Part model, mm, in its own coordinate system. Face numbers are marked on the shaded views. Round coordinates to 2 decimals unless told otherwise and drop trailing zeros. Write each loop counter-clockwise with the first axis right and the second up, starting at its lowest first coordinate (ties: lowest second). Pieces come first, ordered by that corner, then holes.
1) Saw through at C-C on y = 7. Write the cut outline in (x, z), and give its area (3 significant figures).
2) Pull direction X, two halves, no side cores. Call the marked faces 1, 2 and 3: +X half, -X half, draft (parallel to the pull), parting line (faces both ways), or undercut.
3) Saw through at B-B on x = 0. Write the cut outline in (y, z).
4) Drill centre lines: L1, parallel to Y at x = 1, z = -0.5; L2, parallel to X at y = 10.25, z = 1.25; L3, parallel to X at y = 10.25, z = -2. Where is each one in solid material? Low to high.
5) Saw through at A-A on y = 9.5. Write the cut outline in (x, z), and give its area (3 significant figures).
6) Flat gauge pins, fed straight in: pin 1 (3 mm diameter, centred on x = 3.5, y = 9.5, fed in from -Z); pin 2 (2.5 mm diameter, centred on x = 0, y = 11, fed in from +Z); pin 3 (1 mm diameter, centred on y = 6.5, z = 1, fed in from -X). Where does each tip first touch, or does it go through?
```python
from build123d import *
from OCP.BRepFilletAPI import BRepFilletAPI_MakeChamfer

# Parameters (mm, degrees)
BOSS_EXTRUDE1_DEPTH  = 1.75
BOSS_EXTRUDE2_DEPTH  = 0.5
BOSS_EXTRUDE5_DEPTH  = 3.5
SKETCH4_R            = 3.5
BOSS_EXTRUDE7_DEPTH  = 2
SKETCH11_R           = 4.505443821
SKETCH11_R_2         = 3.5
CUT_EXTRUDE3_DEPTH   = 2
SKETCH12_R           = 3.5
CUT_EXTRUDE4_DEPTH   = 3
BOSS_EXTRUDE8_DEPTH  = 2.5
CHAMFER1_SIZE        = 0.5
CHAMFER1_SIZE2       = 0.288675135
SKETCH17_R           = 3.25
BOSS_EXTRUDE9_DEPTH  = 3
SKETCH18_R           = 1.768100224
CUT_EXTRUDE8_DEPTH   = 2.25
SKETCH20_R           = 5
BOSS_EXTRUDE10_DEPTH = 2
SKETCH21_R           = 5
BOSS_EXTRUDE11_DEPTH = 2
FILLET1_R            = 0.5
SKETCH25_R           = 4.000350088
CUT_EXTRUDE9_DEPTH   = 10
SKETCH26_R           = 4.25
BOSS_EXTRUDE12_DEPTH = 2.1


with BuildPart() as part:
    # Sketch1 → Boss-Extrude1 (new body)
    with BuildSketch(Plane(origin=(0, 0, 0), x_dir=(1, 0, 0), z_dir=(0, 1, 0))):
        Polygon((0.658179307, 0), (0.329089653, 0.57), (-0.329089653, 0.57), (-0.658179307, 0), (-0.329089653, -0.57), (0.329089653, -0.57), align=None)
    extrude(amount=BOSS_EXTRUDE1_DEPTH)

    # Sketch2 → Boss-Extrude2 (add)
    with BuildSketch(Plane(origin=(0, 1.75, 0), x_dir=(1, 0, 0), z_dir=(0, 1, 0))):
        Polygon((0.658179307, 0), (0.558124156, -0.173300605), (4.375, 0), (0.558578548, 0.172513574), align=None)
        Polygon((0, 0.197762982), (0, 0), (0, -0.198641554), (0.558124156, -0.173300605), (0.658179307, 0), (0.558578548, 0.172513574), align=None)
    extrude(amount=BOSS_EXTRUDE2_DEPTH)

    # Sketch3 → Boss-Extrude5 (add)
    with BuildSketch(Plane(origin=(0, 1.75, 0), x_dir=(1, 0, 0), z_dir=(0, 1, 0))):
        Polygon((0.658179307, 0), (0.329089653, 0.57), (-0.329089653, 0.57), (-0.658179307, 0), (-0.329089653, -0.57), (0.329089653, -0.57), align=None)
    extrude(amount=BOSS_EXTRUDE5_DEPTH)

    # Sketch4 → Boss-Extrude7 (add)
    with BuildSketch(Plane(origin=(0, 5.25, 0), x_dir=(1, 0, 0), z_dir=(0, 1, 0))):
        with Locations(Location((0, 0, 0), (0, 0, 270))):
            Circle(SKETCH4_R)
    extrude(amount=BOSS_EXTRUDE7_DEPTH)

    # Sketch11 → Cut-Extrude3 (cut)
    with BuildSketch(Plane(origin=(0, 1.75, 0), x_dir=(-1, 0, 0), z_dir=(0, -1, 0))):
        Circle(SKETCH11_R)
        with Locations(Location((0, 0, 0), (0, 0, 270))):
            Circle(SKETCH11_R_2, mode=Mode.SUBTRACT)
    extrude(amount=-CUT_EXTRUDE3_DEPTH, mode=Mode.SUBTRACT)

    # Sketch12 → Cut-Extrude4 (cut)
    with BuildSketch(Plane(origin=(0, 0, 0), x_dir=(-1, 0, 0), z_dir=(0, -1, 0))):
        with Locations(Location((0, 0, 0), (0, 0, 270))):
            Circle(SKETCH12_R)
    extrude(amount=-CUT_EXTRUDE4_DEPTH, mode=Mode.SUBTRACT)

    # Sketch16 → Boss-Extrude8 (add)
    with BuildSketch(Plane(origin=(0, 3, 0), x_dir=(-1, 0, 0), z_dir=(0, -1, 0))):
        Polygon((0.55, -0.952627944), (1.1, 0), (0.658179307, 0), (0.329089653, -0.57), (-0.329089653, -0.57), (-0.658179307, 0), (-1.1, 0), (-0.55, -0.952627944), align=None)
        Polygon((0.658179307, 0), (1.1, 0), (0.55, 0.952627944), (-0.55, 0.952627944), (-1.1, 0), (-0.658179307, 0), (-0.329089653, 0.57), (0.329089653, 0.57), align=None)
        Polygon((-0.658179307, 0), (0.658179307, 0), (0.329089653, 0.57), (-0.329089653, 0.57), align=None)
        Polygon((0.329089653, -0.57), (0.658179307, 0), (-0.658179307, 0), (-0.329089653, -0.57), align=None)
    extrude(amount=-BOSS_EXTRUDE8_DEPTH)

    # Chamfer1: one chamfer whose edges measure the first distance from different faces: ONE call of the kernel's chamfer builder (chamfer() names one face for all edges)
    chamfer1_edges_1 = [part.edges().sort_by_distance(p)[0] for p in [
        (-0.825, 5.25, -0.476313972),
    ]]
    chamfer1_side_1 = [part.faces().sort_by_distance(p)[0] for p in [
        (-0.825, 4.125, -0.476313972),
    ]]
    chamfer1_edges_2 = [part.edges().sort_by_distance(p)[0] for p in [
        (0, 5.25, -0.952627944),
    ]]
    chamfer1_side_2 = [part.faces().sort_by_distance(p)[0] for p in [
        (0, 4.125, -0.952627944),
    ]]
    chamfer1_edges_3 = [part.edges().sort_by_distance(p)[0] for p in [
        (0.825, 5.25, -0.476313972),
    ]]
    chamfer1_side_3 = [part.faces().sort_by_distance(p)[0] for p in [
        (0.825, 4.125, -0.476313972),
    ]]
    chamfer1_edges_4 = [part.edges().sort_by_distance(p)[0] for p in [
        (0.825, 5.25, 0.476313972),
    ]]
    chamfer1_side_4 = [part.faces().sort_by_distance(p)[0] for p in [
        (0.825, 4.125, 0.476313972),
    ]]
    chamfer1_edges_5 = [part.edges().sort_by_distance(p)[0] for p in [
        (0, 5.25, 0.952627944),
    ]]
    chamfer1_side_5 = [part.faces().sort_by_distance(p)[0] for p in [
        (0, 4.125, 0.952627944),
    ]]
    chamfer1_edges_6 = [part.edges().sort_by_distance(p)[0] for p in [
        (-0.825, 5.25, 0.476313972),
    ]]
    chamfer1_side_6 = [part.faces().sort_by_distance(p)[0] for p in [
        (-0.825, 4.125, 0.476313972),
    ]]
    chamfer1 = BRepFilletAPI_MakeChamfer(part.part.solid().wrapped)
    for e in chamfer1_edges_1:
        chamfer1.Add(CHAMFER1_SIZE, CHAMFER1_SIZE2, e.wrapped, chamfer1_side_1[0].wrapped)  # the first distance lies on this face
    for e in chamfer1_edges_2:
        chamfer1.Add(CHAMFER1_SIZE, CHAMFER1_SIZE2, e.wrapped, chamfer1_side_2[0].wrapped)  # the first distance lies on this face
    for e in chamfer1_edges_3:
        chamfer1.Add(CHAMFER1_SIZE, CHAMFER1_SIZE2, e.wrapped, chamfer1_side_3[0].wrapped)  # the first distance lies on this face
    for e in chamfer1_edges_4:
        chamfer1.Add(CHAMFER1_SIZE, CHAMFER1_SIZE2, e.wrapped, chamfer1_side_4[0].wrapped)  # the first distance lies on this face
    for e in chamfer1_edges_5:
        chamfer1.Add(CHAMFER1_SIZE, CHAMFER1_SIZE2, e.wrapped, chamfer1_side_5[0].wrapped)  # the first distance lies on this face
    for e in chamfer1_edges_6:
        chamfer1.Add(CHAMFER1_SIZE, CHAMFER1_SIZE2, e.wrapped, chamfer1_side_6[0].wrapped)  # the first distance lies on this face
    add(Compound.cast(chamfer1.Shape()), mode=Mode.REPLACE)

    # Sketch17 → Boss-Extrude9 (add)
    with BuildSketch(Plane(origin=(0, 3, 0), x_dir=(-1, 0, 0), z_dir=(0, -1, 0))):
        with Locations(Location((0, 0, 0), (0, 0, 90))):
            Circle(SKETCH17_R)
        Polygon((-2.995914926, 0), (-1.497957463, -2.594538434), (1.497957463, -2.594538434), (2.995914926, 0), (1.497957463, 2.594538434), (-1.497957463, 2.594538434), align=None, mode=Mode.SUBTRACT)
    extrude(amount=-BOSS_EXTRUDE9_DEPTH)

    # Sketch18 → Cut-Extrude8 (cut)
    with BuildSketch(Plane(origin=(0, 3, 0), x_dir=(-1, 0, 0), z_dir=(0, -1, 0))):
        Circle(SKETCH18_R)
    extrude(amount=-CUT_EXTRUDE8_DEPTH, mode=Mode.SUBTRACT)

    # Sketch20 → Boss-Extrude10 (add)
    with BuildSketch(Plane(origin=(0, 7.25, 0), x_dir=(1, 0, 0), z_dir=(0, 1, 0))):
        with Locations(Location((0, 0, 0), (0, 0, 270))):
            Circle(SKETCH20_R)
    extrude(amount=-BOSS_EXTRUDE10_DEPTH)

    # Sketch21 → Boss-Extrude11 (add)
    with BuildSketch(Plane(origin=(0, 7.25, 0), x_dir=(1, 0, 0), z_dir=(0, 1, 0))):
        with Locations(Location((0, 0, 0), (0, 0, 270))):
            Circle(SKETCH21_R)
    extrude(amount=BOSS_EXTRUDE11_DEPTH)

    # Fillet1
    fillet1_edges = [part.edges().sort_by_distance(p)[0] for p in [
        (0, 5.25, -5),
        (0, 9.25, -5),
    ]]
    fillet(fillet1_edges, radius=FILLET1_R)

    # Sketch25 → Cut-Extrude9 (cut)
    with BuildSketch(Plane(origin=(0, 5.25, 0), x_dir=(-1, 0, 0), z_dir=(0, -1, 0))):
        Circle(SKETCH25_R)
    extrude(amount=CUT_EXTRUDE9_DEPTH, mode=Mode.SUBTRACT)

    # Sketch26 → Boss-Extrude12 (add)
    with BuildSketch(Plane(origin=(0, 9.25, 0), x_dir=(1, 0, 0), z_dir=(0, 1, 0))):
        with Locations(Location((0, 0, 0), (0, 0, 270))):
            Circle(SKETCH26_R)
        Polygon((1.662768775, -2.88), (3.325537551, 0), (1.662768775, 2.88), (-1.662768775, 2.88), (-3.325537551, 0), (-1.662768775, -2.88), align=None, mode=Mode.SUBTRACT)
    extrude(amount=BOSS_EXTRUDE12_DEPTH)


solid = part.part
```
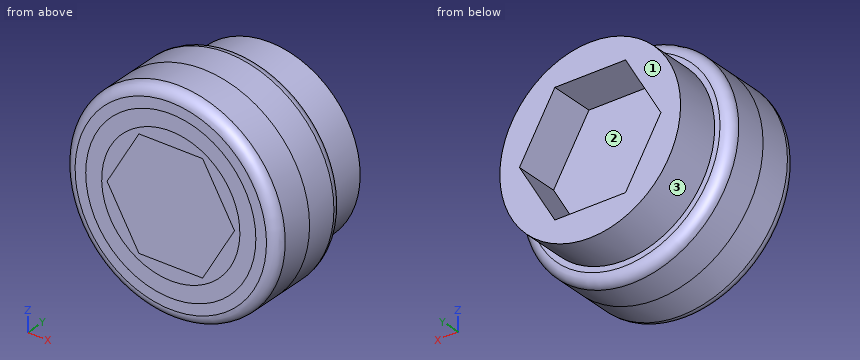
Completed:
1. outline: circle Ø10 at (0, 0)
1. area: 78.5 mm2
2. face 1: draft
2. face 2: undercut
2. face 3: parting line
3. outline: (5.25, -4.5) arc R0.5 ccw to (5.75, -5) - (8.75, -5) arc R0.5 ccw to (9.25, -4.5) - (9.25, -4.25) - (11.35, -4.25) - (11.35, -2.88) - (9.25, -2.88) - (9.25, 2.88) - (11.35, 2.88) - (11.35, 4.25) - (9.25, 4.25) - (9.25, 4.5) arc R0.5 ccw to (8.75, 5) - (5.75, 5) arc R0.5 ccw to (5.25, 4.5) - close
4. L1: y = 5.25 to 9.25
4. L2: x = -4.06 to -2.6, 2.6 to 4.06
4. L3: x = -3.75 to -2.17, 2.17 to 3.75
5. outline: circle Ø8.5 at (0, 0); hole (-3.33, 0) - (-1.66, -2.88) - (1.66, -2.88) - (3.33, 0) - (1.66, 2.88) - (-1.66, 2.88) - close
5. area: 28.0 mm2
6. pin 1: stops at z = -4.5
6. pin 2: stops at z = 4.25
6. pin 3: stops at x = -4.97
